Autodesk Inventor part; units mm, degrees
ref_plane "Work Plane1" through (124.725, 49.8, -24.875) normal (0, 1, 0) x (0, 0, 1)
ref_plane "YZ Plane" through (0, 0, 0) normal (1, 0, 0) x (0, 1, 0)
ref_plane "XZ Plane" through (0, 0, 0) normal (0, 1, 0) x (-1, 0, 0)
sketch "Sketch1" plane through (0, 0, 0) normal (0, 1, 0) x (-1, 0, 0)
  line L0 (-155.225, -15) -> (-155.225, 15)
  line L1 (-155.225, 15) -> (-147.725, 15)
  line L2 (-147.725, 15) -> (-147.725, -15)
  line L3 (-147.725, -15) -> (-155.225, -15)
  circle A0 centre (-171.5, -21.9) radius 1.875
  circle A1 centre (-127.7, 21.9) radius 1.875
  circle A2 centre (-127.7, -21.9) radius 1.875
  circle A3 centre (-171.5, 21.9) radius 1.875
  circle A4 centre (-135.2, 20.8) radius 2.0734
  circle A5 centre (-164, -20.8) radius 2.0734
  circle A6 centre (-135.2, -20.8) radius 2.0734
  circle A7 centre (-128.8, -14.4) radius 2.0734
  circle A8 centre (-128.8, 14.4) radius 2.0734
  circle A9 centre (-164, 20.8) radius 2.0734
  circle A10 centre (-170.4, -14.4) radius 2.0734
  circle A11 centre (-170.4, 14.4) radius 2.0734
  line L4 (-172.5, 24.875) -> (-126.7, 24.875)
  arc A12 (-172.5, 24.875) -> (-174.475, 22.9) centre (-172.5, 22.9) ccw
  line L5 (-174.475, -22.9) -> (-174.475, 22.9)
  arc A13 (-174.475, -22.9) -> (-172.5, -24.875) centre (-172.5, -22.9) ccw
  line L6 (-126.7, -24.875) -> (-172.5, -24.875)
  arc A14 (-126.7, -24.875) -> (-124.725, -22.9) centre (-126.7, -22.9) ccw
  line L7 (-124.725, 22.9) -> (-124.725, -22.9)
  arc A15 (-124.725, 22.9) -> (-126.7, 24.875) centre (-126.7, 22.9) ccw
  point P0 (0, 0)
ref_plane "Work Plane1" through (124.725, 49.8, -24.875) normal (0, 1, 0) x (0, 0, 1)
extrude "Extrusion1" add sketch "Sketch1" along normal blind 4 from surface at 49.8 contours L0 L1 L2 L3 | A0 | A1 | A2 | A3 | L4 A15 L7 A14 L6 A13 L5 A12
properties part number "Outer Cover Top"
Here's how the part is built. I have some questions about the finished solid (model axes, mm). Give positions to 0.01 mm unless a question says otherwise; leave off trailing zeros. Write each loop counter-clockwise with the first axis right and the second up, starting at its lowest first coordinate (ties: lowest second). Pieces come first, ordered by that corner, then holes. Notation, with made-up numbers: M 39,-36.5 L 92,-36.5 A24 ccw 92,-2.5 Z; hole C 73.5,74 d10. An arc over 180 degrees is marked long. Put each result on its own line as item: value. Start each with the question number.
Item 1: If we section it at A-A, the plane x = 135.2: Write out the boundary of the cut face in (y, z) (3 decimals).
Item 2: If we section it at B-B, the plane z = 20.8: Write out the boundary of the cut face in (x, y) (3 decimals), then the cut area to 3 significant figures.
Item 3: If we section it at C-C, the plane y = 52.8: Count the separate pieces of the cut face and the enclosed holes in it, then the cut area to 3 significant figures.
Item 4: I need wall thicknesses on L1, parallel to Z at x = 164, y = 52.5 (3 decimals); L2, parallel to Z at x = 170.4, y = 52.4 (3 decimals); L3, parallel to X at y = 53.2, z = 20.5 (3 decimals). Which ranges of each line are inside material? Lowest first, please. Write a range as from..to.
Values:
1. outline: M 49.8,-24.875 L 53.8,-24.875 L 53.8,-22.873 L 49.8,-22.873 Z; M 49.8,-18.727 L 53.8,-18.727 L 53.8,18.727 L 49.8,18.727 Z; M 49.8,22.873 L 53.8,22.873 L 53.8,24.875 L 49.8,24.875 Z
2. outline: M 124.725,49.8 L 133.127,49.8 L 133.127,53.8 L 124.725,53.8 Z; M 137.273,49.8 L 161.927,49.8 L 161.927,53.8 L 137.273,53.8 Z; M 166.073,49.8 L 174.475,49.8 L 174.475,53.8 L 166.073,53.8 Z
2. area: 166 mm²
3. separate pieces: 1
3. enclosed holes: 8
3. area: 2,360 mm²
4. L1: -24.875..-22.873, -18.727..18.727, 22.873..24.875
4. L2: -24.875..-16.473, -12.327..12.327, 16.473..24.875
4. L3: 124.725..133.148, 137.252..161.948, 166.052..174.475
